from build123d import *

# Parameters (mm, degrees)
F0_R          = 3.175
F0_W          = 5.842
F0_H          = 12.7
F2_DEPTH      = 2.54
F3_R          = 1.524
F4_DEPTH      = 7.62
F4_DEPTH_BACK = 1.27
F5_R          = 1.524
F6_DEPTH      = 17.78


with BuildPart() as f1:
    # F0 (on Front) → F1 (revolve)
    with BuildSketch(Plane.XZ):
        Polygon((5.842, 12.7), (5.842, 0), (66.294, 0), (66.294, 12.7), (56.134, 12.7), (56.134, 10.16), (10.16, 10.16), (10.16, 12.7), align=None)
    revolve(axis=Axis((33.147, 0, 0), (-1, 0, 0)))

    # F0 (on Front) → F2 (join, symmetric)
    with BuildSketch(Plane.XZ):
        with BuildLine():
            Line((5.842, 0), (0, 0))
            Line((0, 0), (-0.9398, 0))
            ThreePointArc((-0.9398, 0), (-3.1957909266, -4.5493385486), (-8.1826630726, -5.5069827884))
            Line((-8.1826630726, -5.5069827884), (5.842, -9.398))
            Line((5.842, -9.398), (5.842, 0))
        make_face()
        with BuildLine():
            ThreePointArc((-8.1826630726, -5.5069827884), (-3.1957909266, -4.5493385486), (-0.9398, 0))
            ThreePointArc((-0.9398, 0), (-4.5919612295, 5.3297205562), (-10.8806298187, 3.8475430269))
            ThreePointArc((-10.8806298187, 3.8475430269), (-12.1459778134, -1.5837270034), (-8.1826630726, -5.5069827884))
        make_face()
        with Locations((-6.6548, 0)):
            Circle(F0_R, mode=Mode.SUBTRACT)
        with BuildLine():
            Line((-0.9398, 0), (0, 0))
            Line((0, 0), (0, 12.7))
            Line((0, 12.7), (5.842, 12.7))
            Line((5.842, 12.7), (5.842, 15.24))
            Line((5.842, 15.24), (-0.508, 15.24))
            Line((-0.508, 15.24), (-10.8806298187, 3.8475430269))
            ThreePointArc((-10.8806298187, 3.8475430269), (-4.5919612295, 5.3297205562), (-0.9398, 0))
        make_face()
        with Locations((2.921, 6.35)):
            Rectangle(F0_W, F0_H)
    extrude(amount=F2_DEPTH, both=True)

    # F3 (on face) → F4 (join, two sides)
    with BuildSketch(Plane.YZ.offset(66.294)) as f4_sk:
        with BuildLine():
            ThreePointArc((-5.08, 0), (0, -5.08), (5.08, 0))
            ThreePointArc((5.08, 0), (0, 5.08), (-5.08, 0))
        make_face()
        Circle(F3_R, mode=Mode.SUBTRACT)
        with BuildLine():
            ThreePointArc((-5.08, 0), (0, 5.08), (5.08, 0))
            Line((5.08, 0), (5.08, 11.6397422652))
            ThreePointArc((5.08, 11.6397422652), (0, 12.7), (-5.08, 11.6397422652))
            Line((-5.08, 11.6397422652), (-5.08, 0))
        make_face()
        with BuildLine():
            ThreePointArc((-5.08, 11.6397422652), (0, 12.7), (5.08, 11.6397422652))
            Line((5.08, 11.6397422652), (5.08, 15.24))
            Line((5.08, 15.24), (-5.08, 15.24))
            Line((-5.08, 15.24), (-5.08, 11.6397422652))
        make_face()
    extrude(amount=F4_DEPTH)
    extrude(f4_sk.sketch, amount=-F4_DEPTH_BACK)

    # F5 (on face) → F6 (cut)
    with BuildSketch(Plane.XY.offset(15.24)):
        with Locations((2.667, 0)):
            Circle(F5_R)
        with Locations((69.5054605603, -0.0776998204)):
            Circle(F5_R)
    extrude(amount=-F6_DEPTH, mode=Mode.SUBTRACT)


solid = f1.part
Geometry check sheet. Reference: the model listing, model coordinates, mm. A direction names the side the tool comes from. Round coordinates to 2 decimals unless told otherwise and drop trailing zeros. Order: outer loops, then holes, each group sorted by start corner. A loop starts at its lowest first (then second) coordinate and runs counter-clockwise, first axis right, second up. Notation, with made-up numbers: M 85,64.25 L 104,64.25 A17 cw 104,76.25 Z; hole C 20,83.5 d3. An arc over 180 degrees is marked long. Answer in a Markdown table with one row per item. Add a question column.
Item 1: Sectioned sample at B-B, the plane x = 58. Enter the section's corners in (y, z).
Item 2: Sectioned sample at A-A, the plane z = 8.75. Enter the section's corners in (x, y), plus the area to 3 significant figures.
Item 3: Set-up check for faces 5 (the face through (-1, -2.54, 3)), 6 (the face through (70.051, 1.454, 0.458)), 7 (the face through (32.825, 10.074, -1.323)): record each of +Z, -Z, +X, -X, +Y, -Y from which the full face is reachable in a straight line by a thin tool's end or side.
Item 4: Sectioned sample at C-C, the plane y = 8. Enter the section's corners in (x, z), plus the area to 3 significant figures.
Item 5: Draft check along Y on faces 1 (the face through (70, 5.08, 8)), 2 (the face through (69, 0, -2.54)), 3 (the face through (65.024, 0, 14)), 4 (the face through (3, 0, -2.54)). Enter one of: released by +Y, released by -Y, zero draft, split by the parting line, or undercut.
Item 6: Sectioned sample at D-D, the plane x = 25. Enter the section's corners in (y, z).
Item 7: Depth check by flat-ended pin: pin 1 Ø6 at (x, y) = (20.5, 6) entering from -Z; pin 2 Ø9 at (x, z) = (-6, 9) entering from +Y; pin 3 Ø5.5 at (x, z) = (-5, 1.5) entering from -Y. Enter the tip coordinate at first touch or a pass-through.
Item 8: Material ranges on L1, parallel to X at y = -8.75, z = 8; L2, parallel to X at y = -7, z = -2.5; L3, parallel to X at y = -5, z = 5, recorded low to high. Write a range as [from, to].
Filled in:
| question | item | result |
|---|---|---|
| 1 | outline | C 0,0 d25.4 |
| 2 | outline | M -6.42,-2.54 L 5.84,-2.54 L 5.84,-9.2 L 10.16,-9.2 L 10.16,-5.16 L 56.13,-5.16 L 56.13,-9.2 L 66.29,-9.2 L 66.29,-5.08 L 73.91,-5.08 L 73.91,5.08 L 66.29,5.08 L 66.29,9.2 L 56.13,9.2 L 56.13,5.16 L 10.16,5.16 L 10.16,9.2 L 5.84,9.2 L 5.84,2.54 L -6.42,2.54 Z; hole C 2.67,0 d3.05; hole C 69.51,-0.08 d3.05 |
| 2 | area | 866 mm² |
| 3 | face 5 | +Z, -Z, -X, -Y |
| 3 | face 6 | +X |
| 3 | face 7 | none |
| 4 | outline | M 5.84,-9.86 L 10.16,-9.86 L 10.16,-6.26 L 56.13,-6.26 L 56.13,-9.86 L 66.29,-9.86 L 66.29,9.86 L 56.13,9.86 L 56.13,6.26 L 10.16,6.26 L 10.16,9.86 L 5.84,9.86 Z |
| 4 | area | 861 mm² |
| 5 | face 1 | released by +Y |
| 5 | face 2 | undercut |
| 5 | face 3 | zero draft |
| 5 | face 4 | undercut |
| 6 | outline | C 0,0 d20.32 |
| 7 | pin 1 | stops at z = -9.71 |
| 7 | pin 2 | stops at y = 2.54 |
| 7 | pin 3 | stops at y = -2.54 |
| 8 | L1 | x = [5.84, 10.16], [56.13, 66.29] |
| 8 | L2 | x = [5.84, 66.29] |
| 8 | L3 | x = [5.84, 73.91] |
